Geometry: see drawing. Coordinates: mm, zero at the bounding-box minimum. Round coordinates to 2 decimals unless told otherwise and drop trailing zeros. Write each loop counter-clockwise with the first axis right and the second up, starting at its lowest first coordinate (ties: lowest second). Pieces come first, ordered by that corner, then holes. Notation, with made-up numbers: (31, 41) - (54, 41) arc R26 ccw to (54, 71) - close; hole circle Ø3 at (48.25, 4). An arc over 180 degrees is marked (long way). One line per item, written item: value. Start each with the question number.
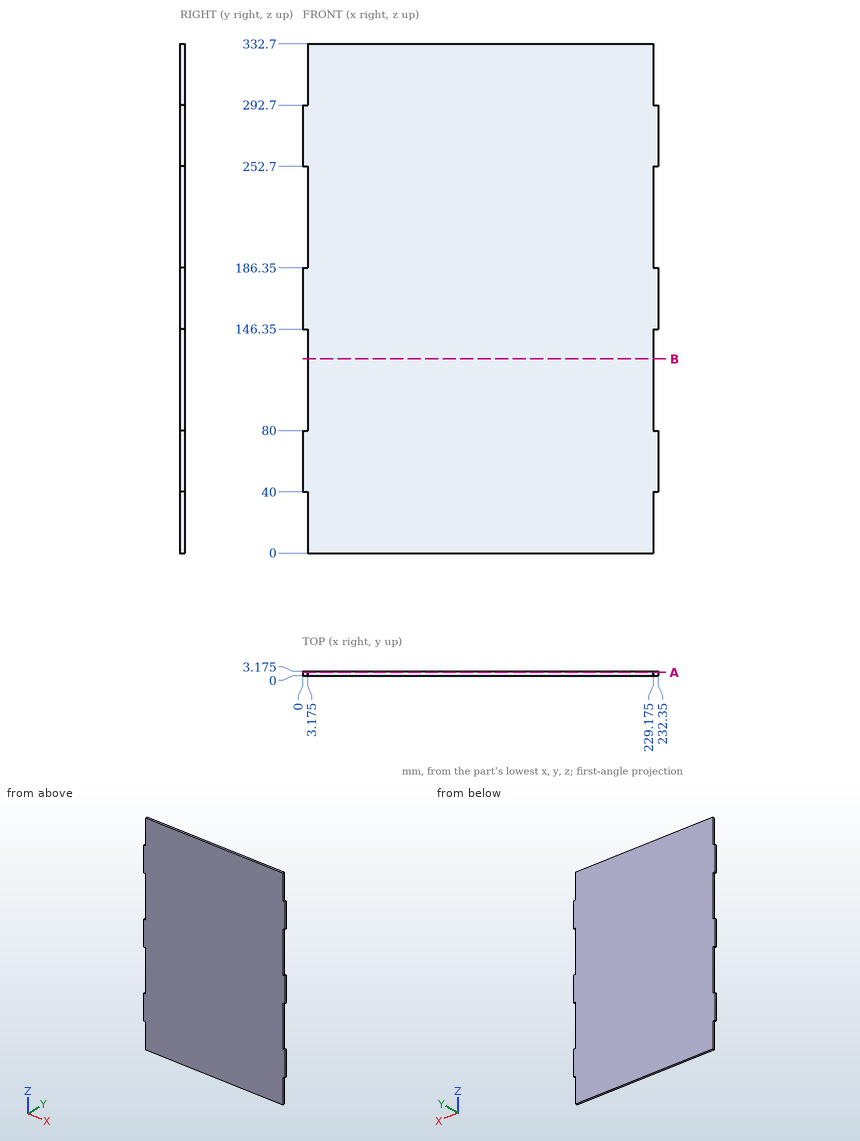
Q1. Cut plane B-B, the plane z = 127. Output: boundary loops of the cut face in (x, y) (3 decimals).
Q2. Material intervals for probe 1 along X at (y, z) = (2.5, 315) (3 decimals), sorted ascending. Write a range as from..to.
Q3. Cut plane A-A, the plane y = 2.4. Output: boundary loops of the cut face in (x, z) (3 decimals), and give its area (3 significant figures).
Q4. Contact query for flat-ended pins moving along their axis: pin 1 Ø1 at (y, z) = (1, 215.5) entering from -X (3 decimals); pin 2 Ø1.6 at (x, y) = (2, 1) entering from +Z; pin 3 Ø1 at (x, y) = (230.5, 1.5) entering from -Z. Output: stop coordinate, or through.
A:
1. outline: (3.175, 0) - (229.175, 0) - (229.175, 3.175) - (3.175, 3.175) - close
2. probe 1: x = 3.175..229.175
3. outline: (0, 40) - (3.175, 40) - (3.175, 0) - (229.175, 0) - (229.175, 40) - (232.35, 40) - (232.35, 80) - (229.175, 80) - (229.175, 146.35) - (232.35, 146.35) - (232.35, 186.35) - (229.175, 186.35) - (229.175, 252.7) - (232.35, 252.7) - (232.35, 292.7) - (229.175, 292.7) - (229.175, 332.7) - (3.175, 332.7) - (3.175, 292.7) - (0, 292.7) - (0, 252.7) - (3.175, 252.7) - (3.175, 186.35) - (0, 186.35) - (0, 146.35) - (3.175, 146.35) - (3.175, 80) - (0, 80) - close
3. area: 76,000 mm²
4. pin 1: stops at x = 3.175
4. pin 2: stops at z = 292.7
4. pin 3: stops at z = 40
